Source: CAD feature listing. Evaluate the final solid. Frame: model axes, mm. A direction names the side the tool comes from. Give positions to 0.01 mm unless a question says otherwise; leave off trailing zeros. Order: outer loops, then holes, each group sorted by start corner. A loop starts at its lowest first (then second) coordinate and runs counter-clockwise, first axis right, second up.
```python
from build123d import *

# Parameters (mm, degrees)
SKETCH_1_W               = 100
SKETCH_1_H               = 50
SKETCH_1_W_2             = 50
SKETCH_1_H_2             = 30
EXTRUDE_1_DEPTH          = 50
SKETCH_2_R               = 14.373245618
EXTRUDE_2_DEPTH          = 30
CUT_EXTRUDE_2_DEPTH      = 154.378616502
CUT_EXTRUDE_2_DEPTH_BACK = 154.378616502
SKETCH_4_W               = 100
SKETCH_4_H               = 50
SKETCH_5_R               = 10
EXTRUDE_3_DEPTH          = 30
SKETCH_6_R               = 14.373245618
EXTRUDE_4_DEPTH          = 10


with BuildPart() as part:
    # 草图1 → 凸台-拉伸1 (new, symmetric)
    with BuildSketch(Plane.XY):
        Rectangle(SKETCH_1_W, SKETCH_1_H)
        with Locations((0, -40)):
            Rectangle(SKETCH_1_W_2, SKETCH_1_H_2)
        Polygon((25, -55), (-25, -55), (-50, -55), (-50, -105), (50, -105), (50, -55), align=None)
    extrude(amount=EXTRUDE_1_DEPTH, both=True)

    # 草图2 → 凸台-拉伸2 (add)
    with BuildSketch(Plane(origin=(0, 0, -50), x_dir=(-1, 0, 0), z_dir=(0, 0, -1))):
        with Locations(Location((0, 0, 0), (0, 0, 180))):
            Circle(SKETCH_2_R)
    extrude(amount=EXTRUDE_2_DEPTH)

    # 草图4 → 切除-拉伸2 (cut, two sides: drawn at the far end of the back side and taken through both)
    with BuildSketch(Plane(origin=(0, 0, -50), x_dir=(-1, 0, 0), z_dir=(0, 0, -1)).offset(-CUT_EXTRUDE_2_DEPTH_BACK)):
        with Locations((0, -80)):
            Rectangle(SKETCH_4_W, SKETCH_4_H)
    extrude(amount=CUT_EXTRUDE_2_DEPTH + CUT_EXTRUDE_2_DEPTH_BACK, mode=Mode.SUBTRACT)

    # 草图5 → 凸台-拉伸3 (add)
    with BuildSketch(Plane(origin=(0, 0, -80), x_dir=(-1, 0, 0), z_dir=(0, 0, -1))):
        Circle(SKETCH_5_R)
    extrude(amount=EXTRUDE_3_DEPTH)

    # 草图6 → 凸台-拉伸4 (add)
    with BuildSketch(Plane(origin=(0, 0, -80), x_dir=(-1, 0, 0), z_dir=(0, 0, -1))):
        with Locations(Location((0, 0, 0), (0, 0, 180))):
            Circle(SKETCH_6_R)
    extrude(amount=EXTRUDE_4_DEPTH)


solid = part.part
```
1) Section query B-B, the plane x = 0. Return the cut outline in (y, z).
Report:
outline: (-55, -50) - (-14.37, -50) - (-14.37, -90) - (-10, -90) - (-10, -110) - (10, -110) - (10, -90) - (14.37, -90) - (14.37, -50) - (25, -50) - (25, 50) - (-55, 50) - close
2) Reachability of faces 1 (the flat face through (25, -40, 1)), 2 (the flat face through (-1, -6, 50)), 3 (the flat face through (-25, -40, 1)), 4 (the cylindrical face through (6.632, 12.752, -69.72)), 5 (the flat face through (50, 0, 1)) from +Z, -Z, +X, -X, +Y, -Y: full face, straight path, thin tool, end or side. Return the list, or none.
Report:
face 1: +Z, -Z, +X, -Y
face 2: +Z, +X, -X, +Y, -Y
face 3: +Z, -Z, -X, -Y
face 4: -Z
face 5: +Z, -Z, +X, +Y, -Y
3) Pin query (flat end, axial travel): pin 1 (12.5 mm diameter, centred on x = -36.5, z = -1.5, fed in from -Y); pin 2 (9 mm diameter, centred on y = -40, z = -14.5, fed in from -X); pin 3 (2 mm diameter, centred on x = -35.5, y = 16.5, fed in from -Z). Return the tip coordinate at first contact, or that it passes through.
Report:
pin 1: stops at y = -25
pin 2: stops at x = -25
pin 3: stops at z = -50
4) Section query A-A, the plane z = -44.5. Return the cut outline in (x, y), and give its area (3 significant figures).
Report:
outline: (-50, -25) - (-25, -25) - (-25, -55) - (25, -55) - (25, -25) - (50, -25) - (50, 25) - (-50, 25) - close
area: 6,500 mm2
5) Material intervals for L1, parallel to Z at x = -37.5, y = -16; L2, parallel to X at y = -39, z = 10; L3, parallel to Z at x = -9, y = -8, sorted ascending.
Report:
L1: z = -50 to 50
L2: x = -25 to 25
L3: z = -90 to 50
6) Section query C-C, the plane y = 0. Return the cut outline in (x, z), and give its area (3 significant figures).
Report:
outline: (-50, -50) - (-14.37, -50) - (-14.37, -90) - (-10, -90) - (-10, -110) - (10, -110) - (10, -90) - (14.37, -90) - (14.37, -50) - (50, -50) - (50, 50) - (-50, 50) - close
area: 11,500 mm2
7) Section query D-D, the plane x = 19. Return the cut outline in (y, z).
Report:
outline: (-55, -50) - (25, -50) - (25, 50) - (-55, 50) - close
